Design review of the part shown in the three views and the two pictorial views. Dimensions are in mm from the part's minimum x, y and z. A direction names the side the tool comes from. Give positions to 0.01 mm unless a question says otherwise; leave off trailing zeros. Loops run counter-clockwise (first coordinate to the right, second up) from the corner with the lowest first, then second, coordinate; pieces in that order, holes last. Notation, with made-up numbers: M 52,-22.75 L 59,-22.75 A23 cw 59,-9.75 Z; hole C -25,39 d5. An arc over 180 degrees is marked long. Return JSON: item names as keys, results as strings. Group by question number.
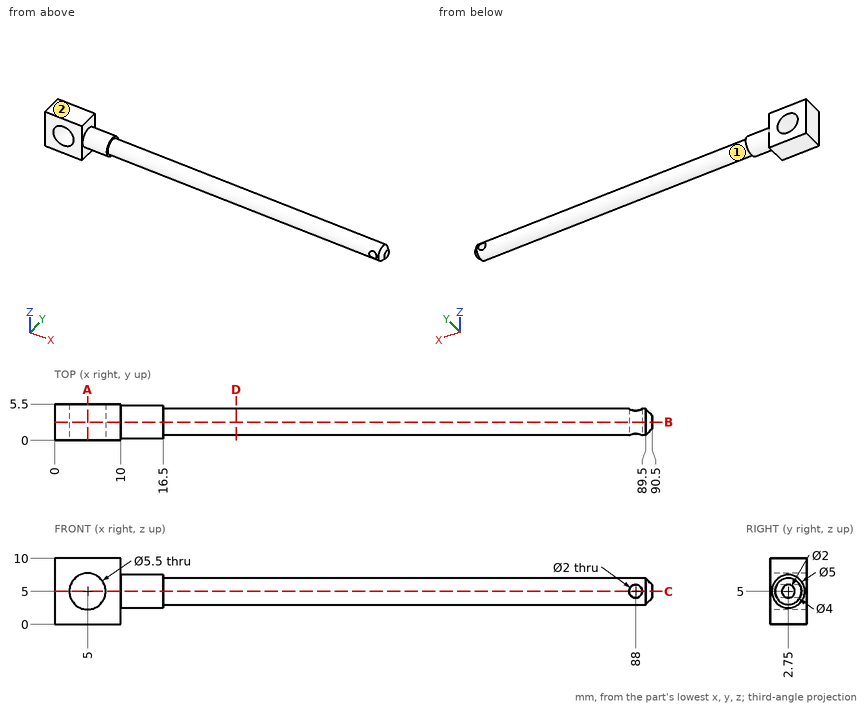
(1) Add section C-C (z = 5). Write out the cut boundary in (x, y).
(2) For probe 1 along X at (y, z) = (2.4, 5); probe 2 along Z at (x, y) = (88, 2.9); probe 3 along X at (y, z) = (3.8, 5), list the stretches that pass through material, from the lowest coordinate up.
(3) Add section D-D (x = 27.5). Write out the cut boundary in (y, z).
(4) Add section B-B (y = 2.75). Write out the cut boundary in (x, z).
(5) For the marked faces 1 and 2, list the 3-axis set-ups (+Z, -Z, +X, -X, +Y, -Y) from which the entire face can be reached by the end or side of a thin tool; tool diameter is ignored.
(6) For pin 1 (1.5 mm diameter, centred on x = 39, y = 0.5, fed in from +Z); pin 2 (2 mm diameter, centred on x = 39.5, z = 8.5, fed in from -Y); pin 3 (1.6 mm diameter, centred on y = 2, z = 2.5, fed in from +X); pin 4 (3 mm diameter, centred on y = 0.5, z = 2.5, fed in from +X), all flat-tipped, find the tip position at first contact; note any pin that passes through.
(7) Add section A-A (x = 5). Write out the cut boundary in (y, z).
Verdict:
{
 "1": {"outline": "M 0,0 L 2.25,0 L 2.25,5.5 L 0,5.5 Z; M 7.75,0 L 10,0 L 10,0.25 L 16.5,0.25 L 16.5,0.75 L 87,0.75 L 87,4.75 L 16.5,4.75 L 16.5,5.25 L 10,5.25 L 10,5.5 L 7.75,5.5 Z; M 89,0.75 L 89.5,0.75 L 90.5,1.75 L 90.5,3.75 L 89.5,4.75 L 89,4.75 Z"},
 "2": {"probe 1": "x = 0 to 2.25, 7.75 to 87, 89 to 90.5", "probe 2": "z = 3.01 to 4, 6 to 6.99", "probe 3": "x = 0 to 2.25, 7.75 to 87, 89 to 90.45"},
 "3": {"outline": "C 2.75,5 d4"},
 "4": {"outline": "M 0,0 L 10,0 L 10,2.5 L 16.5,2.5 L 16.5,3 L 89.5,3 L 90.5,4 L 90.5,6 L 89.5,7 L 16.5,7 L 16.5,7.5 L 10,7.5 L 10,10 L 0,10 Z; hole C 5,5 d5.5; hole C 88,5 d2"},
 "5": {"face 1": "+X", "face 2": "+Z, +X, -X, +Y, -Y"},
 "6": {"pin 1": "stops at z = 6.32", "pin 2": "passes through", "pin 3": "stops at x = 89.69", "pin 4": "stops at x = 89.64"},
 "7": {"outline": "M 0,0 L 5.5,0 L 5.5,2.25 L 0,2.25 Z; M 0,7.75 L 5.5,7.75 L 5.5,10 L 0,10 Z"}
}
